```python
from build123d import *

# Parameters (mm, degrees)
F1_DEPTH = 6.35
F2_R     = 3.175
F3_DEPTH = 6.35
F4_R     = 12.7
F6_DEPTH = 6.35


with BuildPart() as f1:
    # F0 (on Top) → F1 (new body)
    with BuildSketch(Plane.XY):
        Polygon((33.0118411373, 101.6), (-33.0118411373, 101.6), (-86.4261221286, 62.792253257), (-106.8285619826, 0), (-86.4261221286, -62.792253257), (-33.0118411373, -101.6), (33.0118411373, -101.6), (86.4261221286, -62.792253257), (106.8285619826, 0), (86.4261221286, 62.792253257), align=None)
    extrude(amount=F1_DEPTH)

    # F2 (on face) → F3 (cut, through all)
    with BuildSketch(Plane.XY.offset(6.35)):
        with Locations((-30.4149976714, 93.6077376164)):
            Circle(F2_R)
        with Locations((-79.6274976714, 57.8527634569)):
            Circle(F2_R)
        with Locations((-98.425, 0)):
            Circle(F2_R)
        with Locations((-79.6274976714, -57.8527634569)):
            Circle(F2_R)
        with Locations((-30.4149976714, -93.6077376164)):
            Circle(F2_R)
        with Locations((30.4149976714, -93.6077376164)):
            Circle(F2_R)
        with Locations((79.6274976714, -57.8527634569)):
            Circle(F2_R)
        with Locations((98.425, 0)):
            Circle(F2_R)
        with Locations((79.6274976714, 57.8527634569)):
            Circle(F2_R)
        with Locations((30.4149976714, 93.6077376164)):
            Circle(F2_R)
    extrude(amount=-F3_DEPTH, mode=Mode.SUBTRACT)

    # F4
    f4_edges = [f1.edges().sort_by_distance(p)[0] for p in [
        (-86.426122, 62.792253, 3.175),
        (-106.828562, 0, 3.175),
        (-86.426122, -62.792253, 3.175),
        (-33.011841, -101.6, 3.175),
        (33.011841, -101.6, 3.175),
        (86.426122, -62.792253, 3.175),
        (106.828562, 0, 3.175),
        (33.011841, 101.6, 3.175),
        (86.426122, 62.792253, 3.175),
        (-33.011841, 101.6, 3.175),
    ]]
    fillet(f4_edges, radius=F4_R)

    # F5 (on face) → F6 (cut, through all)
    with BuildSketch(Plane.XY.offset(6.35)):
        with BuildLine():
            Line((28.8853609951, 101.6), (-28.8853609951, 101.6))
            ThreePointArc((-28.8853609951, 101.6), (0, 95.9129485994), (28.8853609951, 101.6))
        make_face()
        with BuildLine():
            Line((-36.3502336992, 99.1745158286), (-83.0877295666, 65.2177374284))
            ThreePointArc((-83.0877295666, 65.2177374284), (-56.3762166906, 77.5952053975), (-36.3502336992, 99.1745158286))
        make_face()
        with BuildLine():
            Line((-87.7012746194, 58.8677374284), (-105.5534094917, 3.9245158286))
            ThreePointArc((-105.5534094917, 3.9245158286), (-91.2186347625, 29.6387310978), (-87.7012746194, 58.8677374284))
        make_face()
        with BuildLine():
            Line((-105.5534094917, -3.9245158286), (-87.7012746194, -58.8677374284))
            ThreePointArc((-87.7012746194, -58.8677374284), (-91.2186347625, -29.6387310978), (-105.5534094917, -3.9245158286))
        make_face()
        with BuildLine():
            Line((-83.0877295666, -65.2177374284), (-36.3502336992, -99.1745158286))
            ThreePointArc((-36.3502336992, -99.1745158286), (-56.3762166906, -77.5952053975), (-83.0877295666, -65.2177374284))
        make_face()
        with BuildLine():
            Line((-28.8853609951, -101.6), (28.8853609951, -101.6))
            ThreePointArc((28.8853609951, -101.6), (0, -95.9129485994), (-28.8853609951, -101.6))
        make_face()
        with BuildLine():
            Line((36.3502336992, -99.1745158286), (83.0877295666, -65.2177374284))
            ThreePointArc((83.0877295666, -65.2177374284), (56.3762166906, -77.5952053975), (36.3502336992, -99.1745158286))
        make_face()
        with BuildLine():
            Line((87.7012746194, -58.8677374284), (105.5534094917, -3.9245158286))
            ThreePointArc((105.5534094917, -3.9245158286), (91.2186347625, -29.6387310978), (87.7012746194, -58.8677374284))
        make_face()
        with BuildLine():
            Line((105.5534094917, 3.9245158286), (87.7012746194, 58.8677374284))
            ThreePointArc((87.7012746194, 58.8677374284), (91.2186347625, 29.6387310978), (105.5534094917, 3.9245158286))
        make_face()
        with BuildLine():
            Line((83.0877295666, 65.2177374284), (36.3502336992, 99.1745158286))
            ThreePointArc((36.3502336992, 99.1745158286), (56.3762166906, 77.5952053975), (83.0877295666, 65.2177374284))
        make_face()
    extrude(amount=-F6_DEPTH, mode=Mode.SUBTRACT)


solid = f1.part
```
The listing builds one solid part. Answer for the finished solid, in the listing's coordinates (mm). A direction names the side the tool comes from. Coordinates: 2 decimals unless noted, no trailing zeros. Write each loop counter-clockwise with the first axis right and the second up, starting at its lowest first coordinate (ties: lowest second). Pieces come first, ordered by that corner, then holes. Notation, with made-up numbers: (77, 65.5) - (117, 65.5) arc R10 ccw to (117, 80.5) - close; hole circle Ø2 at (59, 26). An arc over 180 degrees is marked (long way). Return JSON: item names as keys, results as strings. Group by question number.
1. Which of the six approach directions +Z, -Z, +X, -X, +Y, -Y give full straight-line access (tool end or side, diameter ignored) to faces 1 (the cylindrical face through (-56.712, 77.352, 3.219)), 2 (the cylindrical face through (-91.092, -30.034, 3.219))?
2. Given pin 1 (1.5 mm diameter, centred on y = 33.5, z = 3.5, fed in from +X); pin 2 (4 mm diameter, centred on x = 79.63, y = 57.85, fed in from +Z), each flat-ended and moving along its own axis, determine where each tip first touches the part or whether it passes through.
3. A cutting plane is placed at D-D, the plane y = -87. Determine the outline of the cut face in (x, z), plus the area to 3 significant figures.
4. A cutting plane is placed at A-A, the plane y = 0. Determine the outline of the cut face in (x, z) (3 decimals), plus the area to 3 significant figures.
5. Determine the mould class of faces 3 (the cylindrical face through (-32.76, 95.75, 3.22)), 4 (the cylindrical face through (56.712, -77.352, 3.219)), 5 (the cylindrical face through (29.7, -96.7, 3.2)), 6 (the cylindrical face through (-0.415, 95.914, 3.219)) for opening direction Y: released by +Y, released by -Y, zero draft, split by the parting line, or undercut.
6. A cutting plane is placed at B-B, the plane z = 2. Give the number of separate pieces and of enclosed holes in the cut face, plus the area to 3 significant figures.
7. Straight lines are drawn through the part: L1, parallel to X at y = 59.5, z = 4.25; L2, parallel to X at y = -91, z = 1.75; L3, parallel to Y at x = 29.5, z = 4. For each, find the intervals that lie inside material, in ascending order.
8. A cutting plane is placed at C-C, the plane x = -6. Determine the outline of the cut face in (y, z), plus the area to 3 significant figures.
Ans:
{
 "1": {"face 1": "+Z, -Z, -X, +Y", "face 2": "+Z, -Z, -X"},
 "2": {"pin 1": "x = 90.28", "pin 2": "through"},
 "3": {"outline": "(-45.69, 0) - (45.69, 0) - (45.69, 6.35) - (-45.69, 6.35) - close", "area": "580 mm²"},
 "4": {"outline": "(-106.175, 0) - (-101.6, 0) - (-101.6, 6.35) - (-106.175, 6.35) - close; (-95.25, 0) - (95.25, 0) - (95.25, 6.35) - (-95.25, 6.35) - close; (101.6, 0) - (106.175, 0) - (106.175, 6.35) - (101.6, 6.35) - close", "area": "1,270 mm²"},
 "5": {"face 3": "undercut", "face 4": "released by -Y", "face 5": "undercut", "face 6": "released by +Y"},
 "6": {"separate pieces": "1", "enclosed holes": "10", "area": "31,000 mm²"},
 "7": {"L1": "-87.48 to -82.34, -76.91 to 76.91, 82.34 to 87.48", "L2": "-42.18 to -32.23, -28.6 to 28.6, 32.23 to 42.18", "L3": "-101.59 to -96.65, -90.57 to 90.57, 96.65 to 101.59"},
 "8": {"outline": "(-96.15, 0) - (96.15, 0) - (96.15, 6.35) - (-96.15, 6.35) - close", "area": "1,220 mm²"}
}
